Can you work these out from the model? Positions are in its coordinate system, mm. A direction names the side the tool comes from. Coordinates: 2 decimals unless noted, no trailing zeros. Order: outer loops, then holes, each group sorted by start corner. A loop starts at its lowest first (then second) coordinate and runs counter-clockwise, first axis right, second up. Notation, with made-up numbers: M -23,20.25 L 14,20.25 A21 ccw 14,51.25 Z; hole C 22,57.5 d7. An arc over 180 degrees is marked long. Answer as a JSON object with one key per item and string values.
from build123d import *

# Parameters (mm, degrees)
SKETCH1_W                      = 118.11
SKETCH1_H                      = 149.86
BASE_FLANGE1_DEPTH             = 2.286
EDGE_FLANGE1_STRIP_W           = 13.716
EDGE_FLANGE1_STRIP_H           = 2.286
EDGE_FLANGE1_STRIP_CUT_DEPTH   = 149.86
EDGE_FLANGE1_STRIP_2_W         = 13.716
EDGE_FLANGE1_STRIP_2_H         = 2.286
EDGE_FLANGE1_STRIP_CUT_2_DEPTH = 149.86
EDGE_FLANGE1_DEPTH             = 149.86
EDGE_FLANGE1_BEND_DEPTH        = 149.86
EDGE_FLANGE10_DEPTH            = 108.966
EDGE_FLANGE10_START            = 2.286
EDGE_FLANGE10_PROFILE_W        = 108.966
EDGE_FLANGE10_PROFILE_H        = 38.354
EDGE_FLANGE10_PROFILE_R        = 3.3734375
EDGE_FLANGE10_FLAT_DEPTH       = 2.286
UNFOLD6_START                  = -42.926
UNFOLD6_OUTLINE_W              = 108.966
UNFOLD6_OUTLINE_H              = 4.572
UNFOLD6_DEPTH                  = 40.64
UNFOLD6_START_2                = -2.286
UNFOLD6_2_OUTLINE_W            = 108.966
UNFOLD6_2_OUTLINE_H            = 43.740260605
UNFOLD6_2_OUTLINE_R            = 3.3734375
UNFOLD6_2_DEPTH                = 2.286
SKETCH121_W                    = 60.325
SKETCH121_H                    = 50.8
CUT_EXTRUDE3_DEPTH             = 134.454815623
EDGE_FLANGE16_DEPTH            = 44.45
FOLD3_START                    = -54.483
FOLD3_DEPTH                    = 108.966
FOLD3_START_2                  = -37.9015624
FOLD3_2_OUTLINE_W              = 2.286
FOLD3_2_OUTLINE_H              = 24.690260605
FOLD3_2_DEPTH                  = 75.8031248
FOLD3_3_DEPTH                  = 9.8345624
FOLD3_START_3                  = 44.6484376
FOLD3_4_DEPTH                  = 9.8345624
FOLD3_5_DEPTH                  = 24.3205
FOLD3_START_4                  = 30.1625
FOLD3_6_DEPTH                  = 24.3205
FOLD3_START_5                  = 77.216
FOLD3_7_DEPTH                  = 2.286
SKETCH128_R                    = 1.5875
CUT_EXTRUDE4_DEPTH             = 109.553505374
FILLET3_R                      = 6.35
SKETCH130_R                    = 3.3734375
CUT_EXTRUDE6_DEPTH             = 150.152078779


with BuildPart() as part:
    # Base-Flange1: sheet metal written as solids
    # Sketch1 → Base-Flange1 (new body)
    with BuildSketch(Plane.XY):
        Rectangle(SKETCH1_W, SKETCH1_H)
    extrude(amount=-BASE_FLANGE1_DEPTH)

    # Edge-Flange1: sheet metal written as solids
    # Edge-Flange1 strip (on a plane across the edge) → Edge-Flange1 strip cut (cut)
    with BuildSketch(Plane(origin=(-59.055, 74.93, 0), x_dir=(1, 0, 0), z_dir=(0, -1, 0))):
        with Locations((-2.286, -1.143)):
            Rectangle(EDGE_FLANGE1_STRIP_W, EDGE_FLANGE1_STRIP_H)
    extrude(amount=EDGE_FLANGE1_STRIP_CUT_DEPTH, mode=Mode.SUBTRACT)

    # Edge-Flange1 strip 2 (on a plane across the edge) → Edge-Flange1 strip cut 2 (cut)
    with BuildSketch(Plane(origin=(59.055, -74.93, 0), x_dir=(-1, 0, 0), z_dir=(0, 1, 0))):
        with Locations((-2.286, -1.143)):
            Rectangle(EDGE_FLANGE1_STRIP_2_W, EDGE_FLANGE1_STRIP_2_H)
    extrude(amount=EDGE_FLANGE1_STRIP_CUT_2_DEPTH, mode=Mode.SUBTRACT)

    # Edge-Flange1 section (on a plane across the edge) → Edge-Flange1 (add)
    with BuildSketch(Plane(origin=(-59.055, 74.93, 0), x_dir=(1, 0, 0), z_dir=(0, -1, 0))):
        with BuildLine():
            Line((0, 2.286), (0, 15.494))
            Line((0, 15.494), (2.286, 15.494))
            Line((2.286, 15.494), (2.286, 2.286))
            ThreePointArc((2.286, 2.286), (2.955553898, 0.669553898), (4.572, 0))
            Line((4.572, 0), (4.572, -2.286))
            ThreePointArc((4.572, -2.286), (1.339107796, -0.946892204), (0, 2.286))
        make_face()
    extrude(amount=EDGE_FLANGE1_DEPTH)

    # Edge-Flange1 section 2 (on a plane across the edge) → Edge-Flange1 bend (add)
    with BuildSketch(Plane(origin=(59.055, -74.93, 0), x_dir=(-1, 0, 0), z_dir=(0, 1, 0))):
        with BuildLine():
            Line((0, 2.286), (0, 15.494))
            Line((0, 15.494), (2.286, 15.494))
            Line((2.286, 15.494), (2.286, 2.286))
            ThreePointArc((2.286, 2.286), (2.955553898, 0.669553898), (4.572, 0))
            Line((4.572, 0), (4.572, -2.286))
            ThreePointArc((4.572, -2.286), (1.339107796, -0.946892204), (0, 2.286))
        make_face()
    extrude(amount=EDGE_FLANGE1_BEND_DEPTH)

    # Edge-Flange10: sheet metal written as solids
    # Edge-Flange10 bend section (on a plane across the edge) → Edge-Flange10 (add)
    with BuildSketch(Plane(origin=(-54.483, 77.216, -2.286), x_dir=(0, -1, 0), z_dir=(1, 0, 0))):
        with BuildLine():
            Line((-2.286, 2.286), (0, 2.286))
            ThreePointArc((0, 2.286), (0.669553898, 0.669553898), (2.286, 0))
            Line((2.286, 0), (2.286, -2.286))
            ThreePointArc((2.286, -2.286), (-0.946892204, -0.946892204), (-2.286, 2.286))
        make_face()
    extrude(amount=EDGE_FLANGE10_DEPTH)

    # Edge-Flange10 profile (on flange) → Edge-Flange10 flat (add)
    with BuildSketch(Plane(origin=(0, 77.216, -2.286), x_dir=(1, 0, 0), z_dir=(0, 1, 0)).offset(EDGE_FLANGE10_START)):
        with Locations((0, 21.463)):
            Rectangle(EDGE_FLANGE10_PROFILE_W, EDGE_FLANGE10_PROFILE_H)
        with Locations((41.275, 22.225)):
            Circle(EDGE_FLANGE10_PROFILE_R, mode=Mode.SUBTRACT)
        with Locations((-41.275, 22.225)):
            Circle(EDGE_FLANGE10_PROFILE_R, mode=Mode.SUBTRACT)
    extrude(amount=-EDGE_FLANGE10_FLAT_DEPTH)

    # Unfold6: read off the stored shape, not the designer's step
    # Unfold6 outline → Unfold6 (cut)
    with BuildSketch(Plane.XY.offset(UNFOLD6_START)):
        with Locations((0, 77.216)):
            Rectangle(UNFOLD6_OUTLINE_W, UNFOLD6_OUTLINE_H)
    extrude(amount=UNFOLD6_DEPTH, mode=Mode.SUBTRACT)

    # Unfold6 2 outline → Unfold6 2 (add)
    with BuildSketch(Plane.XY.offset(UNFOLD6_START_2)):
        with Locations((0, 96.800130303)):
            Rectangle(UNFOLD6_2_OUTLINE_W, UNFOLD6_2_OUTLINE_H)
        with Locations((-41.275, 100.255260605)):
            Circle(UNFOLD6_2_OUTLINE_R, mode=Mode.SUBTRACT)
        with Locations((41.275, 100.255260605)):
            Circle(UNFOLD6_2_OUTLINE_R, mode=Mode.SUBTRACT)
    extrude(amount=UNFOLD6_2_DEPTH)

    # Sketch121 → Cut-Extrude3 (cut, through all)
    with BuildSketch(Plane.XY):
        with Locations((0, 68.58)):
            Rectangle(SKETCH121_W, SKETCH121_H)
    extrude(amount=-CUT_EXTRUDE3_DEPTH, mode=Mode.SUBTRACT)

    # Edge-Flange16: sheet metal written as solids
    # Edge-Flange16 section (on a plane across the edge) → Edge-Flange16 (add)
    with BuildSketch(Plane(origin=(22.225, 45.466, 0), x_dir=(0, -1, 0), z_dir=(-1, 0, 0))):
        with BuildLine():
            Line((-2.286, 2.286), (-2.286, 44.45))
            Line((-2.286, 44.45), (0, 44.45))
            Line((0, 44.45), (0, 2.286))
            ThreePointArc((0, 2.286), (0.669553898, 0.669553898), (2.286, 0))
            Line((2.286, 0), (2.286, -2.286))
            ThreePointArc((2.286, -2.286), (-0.946892204, -0.946892204), (-2.286, 2.286))
        make_face()
    extrude(amount=EDGE_FLANGE16_DEPTH)

    # Fold3: read off the stored shape, not the designer's step
    # Fold3 outline → Fold3 (cut)
    with BuildSketch(Plane.YZ.offset(FOLD3_START)):
        with BuildLine():
            ThreePointArc((74.93, 0), (77.216, -0.612531854), (78.889468147, -2.286))
            Line((78.889468147, -2.286), (118.670260605, -2.286))
            Line((118.670260605, -2.286), (118.670260605, 0))
            Line((118.670260605, 0), (74.93, 0))
        make_face()
    extrude(amount=FOLD3_DEPTH, mode=Mode.SUBTRACT)

    # Fold3 3 outline → Fold3 3 (add)
    with BuildSketch(Plane.YZ.offset(FOLD3_START)):
        with BuildLine():
            ThreePointArc((74.93, -2.286), (76.546446102, -2.955553898), (77.216, -4.572))
            Line((77.216, -4.572), (77.216, -42.926))
            Line((77.216, -42.926), (79.502, -42.926))
            Line((79.502, -42.926), (79.502, -4.572))
            ThreePointArc((79.502, -4.572), (79.346212878, -3.388679326), (78.889468147, -2.286))
            Line((78.889468147, -2.286), (74.93, -2.286))
        make_face()
    extrude(amount=FOLD3_3_DEPTH)

    # Fold3 4 outline → Fold3 4 (add)
    with BuildSketch(Plane.YZ.offset(FOLD3_START_3)):
        with BuildLine():
            ThreePointArc((74.93, -2.286), (76.546446102, -2.955553898), (77.216, -4.572))
            Line((77.216, -4.572), (77.216, -42.926))
            Line((77.216, -42.926), (79.502, -42.926))
            Line((79.502, -42.926), (79.502, -4.572))
            ThreePointArc((79.502, -4.572), (79.346212878, -3.388679326), (78.889468147, -2.286))
            Line((78.889468147, -2.286), (74.93, -2.286))
        make_face()
    extrude(amount=FOLD3_4_DEPTH)



with BuildPart() as body_2:
    # Fold3 2 outline → Fold3 2 (new body)
    with BuildSketch(Plane.YZ.offset(FOLD3_START_2)):
        with Locations((78.359, -30.580869697)):
            Rectangle(FOLD3_2_OUTLINE_W, FOLD3_2_OUTLINE_H)
    extrude(amount=FOLD3_2_DEPTH)


with BuildPart() as part_1:
    add(part.part)

    add(body_2.part)  # Fold3 5 merges body 2
    # Fold3 5 outline → Fold3 5 (add)
    with BuildSketch(Plane.YZ.offset(FOLD3_START)):
        with BuildLine():
            ThreePointArc((74.93, -2.286), (76.546446102, -2.955553898), (77.216, -4.572))
            Line((77.216, -4.572), (77.216, -18.235739395))
            Line((77.216, -18.235739395), (79.502, -18.235739395))
            Line((79.502, -18.235739395), (79.502, -4.572))
            ThreePointArc((79.502, -4.572), (79.346212878, -3.388679326), (78.889468147, -2.286))
            Line((78.889468147, -2.286), (74.93, -2.286))
        make_face()
    extrude(amount=FOLD3_5_DEPTH)

    # Fold3 6 outline → Fold3 6 (add)
    with BuildSketch(Plane.YZ.offset(FOLD3_START_4)):
        with BuildLine():
            ThreePointArc((74.93, -2.286), (76.546446102, -2.955553898), (77.216, -4.572))
            Line((77.216, -4.572), (77.216, -18.235739395))
            Line((77.216, -18.235739395), (79.502, -18.235739395))
            Line((79.502, -18.235739395), (79.502, -4.572))
            ThreePointArc((79.502, -4.572), (79.346212878, -3.388679326), (78.889468147, -2.286))
            Line((78.889468147, -2.286), (74.93, -2.286))
        make_face()
    extrude(amount=FOLD3_6_DEPTH)

    # Fold3 7 outline → Fold3 7 (add)
    with BuildSketch(Plane(origin=(0, 0, 0), x_dir=(1, 0, 0), z_dir=(0, 1, 0)).offset(FOLD3_START_5)):
        with BuildLine():
            Line((44.6484376, 18.235739395), (44.6484375, 24.511))
            ThreePointArc((44.6484375, 24.511), (41.275, 21.1375625), (37.9015625, 24.511))
            Line((37.9015625, 24.511), (37.9015624, 18.235739395))
            Line((37.9015624, 18.235739395), (44.6484376, 18.235739395))
        make_face()
        with BuildLine():
            Line((-37.9015625, 24.511), (-37.9015624, 42.926))
            Line((-37.9015624, 42.926), (-44.6484376, 42.926))
            Line((-44.6484376, 42.926), (-44.6484375, 24.511))
            ThreePointArc((-44.6484375, 24.511), (-41.275, 27.8844375), (-37.9015625, 24.511))
        make_face()
        with BuildLine():
            ThreePointArc((37.9015625, 24.511), (41.275, 27.8844375), (44.6484375, 24.511))
            Line((44.6484375, 24.511), (44.6484376, 42.926))
            Line((44.6484376, 42.926), (37.9015624, 42.926))
            Line((37.9015624, 42.926), (37.9015625, 24.511))
        make_face()
        with BuildLine():
            Line((-37.9015624, 18.235739395), (-37.9015625, 24.511))
            ThreePointArc((-37.9015625, 24.511), (-41.275, 21.1375625), (-44.6484375, 24.511))
            Line((-44.6484375, 24.511), (-44.6484376, 18.235739395))
            Line((-44.6484376, 18.235739395), (-37.9015624, 18.235739395))
        make_face()
    extrude(amount=FOLD3_7_DEPTH)

    # Sketch128 → Cut-Extrude4 (cut, through all)
    with BuildSketch(Plane.XY):
        with Locations((-29.718, 36.957)):
            Circle(SKETCH128_R)
        with Locations((19.812, 36.957)):
            Circle(SKETCH128_R)
        with Locations((19.812, -68.58)):
            Circle(SKETCH128_R)
        with Locations((-29.718, -68.58)):
            Circle(SKETCH128_R)
    extrude(amount=-CUT_EXTRUDE4_DEPTH, mode=Mode.SUBTRACT)

    # Fillet3
    fillet3_edges = [part_1.edges().sort_by_distance(p)[0] for p in [
        (-57.912, 74.93, 15.494),
        (57.912, -74.93, 15.494),
        (-57.912, -74.93, 15.494),
        (-22.225, 46.609, 44.45),
        (22.225, 46.609, 44.45),
        (-54.483, 78.359, -42.926),
        (54.483, 78.359, -42.926),
        (57.912, 74.93, 15.494),
        (30.1625, 78.359, -18.235739395),
        (-30.1625, 78.359, -18.235739395),
        (-30.1625, 43.18, -1.143),
        (30.1625, 43.18, -1.143),
    ]]
    fillet(fillet3_edges, radius=FILLET3_R)

    # Sketch130 → Cut-Extrude6 (cut, through all)
    with BuildSketch(Plane(origin=(59.055, 0, 0), x_dir=(0, 0, -1), z_dir=(1, 0, 0))):
        with Locations((-8.89, -62.23)):
            Circle(SKETCH130_R)
        with Locations((-8.89, 62.23)):
            Circle(SKETCH130_R)
    extrude(amount=-CUT_EXTRUDE6_DEPTH, mode=Mode.SUBTRACT)


solid = part_1.part
Item 1: Which directions (+Z, -Z, +X, -X, +Y, -Y) give clear straight access to the entire face, cutting with the end or side of a thin tool? Please do faces 4 (the flat face through (-57, 74.93, 4)), 5 (the flat face through (-56.769, 1, 9)), 6 (the flat face through (0, 45.466, 24)).
Answers follow:
{"face 4": "+Z, -Z, -X, +Y", "face 5": "+Z, +Y, -Y", "face 6": "+Z, -Y"}
Item 2: I want a section at C-C, the plane y = 62.23. Write out the boundary of the cut face in (x, z) (1 decimal), plus the area to 3 significant figures.
Answers follow:
{"outline": "M -59.1,2.3 A4.6 ccw -54.5,-2.3 L -30.2,-2.3 L -30.2,0 L -54.5,0 A2.3 cw -56.8,2.3 L -56.8,5.5 L -59.1,5.5 Z; M -59.1,12.3 L -56.8,12.3 L -56.8,15.5 L -59.1,15.5 Z; M 30.2,-2.3 L 54.5,-2.3 A4.6 ccw 59.1,2.3 L 59.1,5.5 L 56.8,5.5 L 56.8,2.3 A2.3 cw 54.5,0 L 30.2,0 Z; M 56.8,12.3 L 59.1,12.3 L 59.1,15.5 L 56.8,15.5 Z", "area": "165 mm^2"}
Item 3: If we mould it in two halves opening along Z, with no side actions, what happens to faces 1 (the cylindrical face through (57.928, 58.937, 9.621)), 2 (the cylindrical face through (28.35, 78.38, -16.33)), 3 (the cylindrical face through (-28.35, 45.09, -1.16))? For each: pulls with the +Z half, pulls with the -Z half, needs draft (parallel to the pull), parting line crosses it, or undercut.
Answers follow:
{"face 1": "undercut", "face 2": "pulls with the +Z half", "face 3": "needs draft"}
Item 4: I want a section at B-B, the plane z = -9. Write out the boundary of the cut face in (x, y), plus the area to 3 significant figures.
Answers follow:
{"outline": "M -54.48,77.22 L -30.16,77.22 L -30.16,79.5 L -54.48,79.5 Z; M 30.16,77.22 L 54.48,77.22 L 54.48,79.5 L 30.16,79.5 Z", "area": "111 mm^2"}
Item 5: Please list where these lines run through material, in increasing order: line 1 (Y direction, x = 57.9, z = 8.89); line 2 (Y direction, x = -3, z = -38.5); line 3 (Z direction, x = -28.5, y = 34).
Answers follow:
{"line 1": "y = -74.93 to -65.6, -58.86 to 58.86, 65.6 to 74.93", "line 2": "y = 77.22 to 79.5", "line 3": "z = -2.29 to 0"}
Item 6: I'm going to push flat-ended pins straight in: pin 1 (19 mm diameter, centred on x = -11.5, z = -30, fed in from -Y); pin 2 (4 mm diameter, centred on y = 62.23, z = 8.89, fed in from -X); pin 3 (12.5 mm diameter, centred on x = -8, z = 23, fed in from +Y); pin 4 (5 mm diameter, centred on x = -6, y = -18.5, fed in from +Z). Where does each tip first touch, or does it pass through?
Answers follow:
{"pin 1": "stops at y = 77.22", "pin 2": "passes through", "pin 3": "stops at y = 47.75", "pin 4": "stops at z = 0"}
Item 7: I want a section at D-D, the plane y = -62.23. Write out the boundary of the cut face in (x, z) (3 decimals).
Answers follow:
{"outline": "M -59.055,2.286 A4.572 ccw -54.483,-2.286 L 54.483,-2.286 A4.572 ccw 59.055,2.286 L 59.055,5.517 L 56.769,5.517 L 56.769,2.286 A2.286 cw 54.483,0 L -54.483,0 A2.286 cw -56.769,2.286 L -56.769,5.517 L -59.055,5.517 Z; M -59.055,12.263 L -56.769,12.263 L -56.769,15.494 L -59.055,15.494 Z; M 56.769,12.263 L 59.055,12.263 L 59.055,15.494 L 56.769,15.494 Z"}
Item 8: I want a section at A-A, the plane x = -8. Write out the boundary of the cut face in (y, z), plus the area to 3 significant figures.
Answers follow:
{"outline": "M -74.93,-2.29 L 43.18,-2.29 A4.57 ccw 47.75,2.29 L 47.75,44.45 L 45.47,44.45 L 45.47,2.29 A2.29 cw 43.18,0 L -74.93,0 Z; M 77.22,-42.93 L 79.5,-42.93 L 79.5,-18.24 L 77.22,-18.24 Z", "area": "435 mm^2"}
